from build123d import *

# Parameters (mm, degrees)
CROQUIS2_W              = 92
CROQUIS2_H              = 62
SALIENTE_EXTRUIR1_DEPTH = 8
CROQUIS3_W              = 89
CROQUIS3_H              = 59
CORTAR_EXTRUIR1_DEPTH   = 2
CROQUIS4_W              = 87
CROQUIS4_H              = 57
CORTAR_EXTRUIR2_DEPTH   = 3
CROQUIS5_W              = 10
CROQUIS5_H              = 53.632525493
CORTAR_EXTRUIR3_DEPTH   = 1
CORTAR_EXTRUIR4_REACH   = 57.696
CROQUIS6_W              = 15
CROQUIS6_H              = 10
CROQUIS7_R              = 5
CORTAR_EXTRUIR5_DEPTH   = 56.794264938
REDONDEO1_R             = 5
CROQUIS9_W              = 2.5
CROQUIS9_H              = 17.009234147
CROQUIS9_H_2            = 13.999979608
CROQUIS9_H_3            = 14.150072655
CROQUIS9_W_2            = 9.965409089
CROQUIS9_H_4            = 2.5
CROQUIS9_W_3            = 7.294458122
CROQUIS9_W_4            = 7.420347284
CROQUIS9_W_5            = 5
CORTAR_EXTRUIR7_DEPTH   = 2
CROQUIS10_R             = 1.492354092
CROQUIS10_R_2           = 1.54105633
CROQUIS10_R_3           = 1.454647155
CROQUIS10_R_4           = 1.436117112
CORTAR_EXTRUIR8_DEPTH   = 56.695601345
CORTAR_EXTRUIR9_REACH   = 99.411
CROQUIS11_W             = 15
CROQUIS11_H             = 8
CROQUIS12_W             = 50.407466657
CROQUIS12_H             = 2
CORTAR_EXTRUIR10_DEPTH  = 2.5
CROQUIS13_W             = 52.657281968
CROQUIS13_H             = 2
CORTAR_EXTRUIR11_DEPTH  = 2.5


with BuildPart() as part:
    # Croquis2 → Saliente-Extruir1 (new body)
    with BuildSketch(Plane(origin=(0, 0, 0), x_dir=(1, 0, 0), z_dir=(0, 1, 0))):
        Rectangle(CROQUIS2_W, CROQUIS2_H)
    extrude(amount=SALIENTE_EXTRUIR1_DEPTH)

    # Croquis3 → Cortar-Extruir1 (cut)
    with BuildSketch(Plane(origin=(0, 8, 0), x_dir=(1, 0, 0), z_dir=(0, 1, 0))):
        Rectangle(CROQUIS3_W, CROQUIS3_H)
    extrude(amount=-CORTAR_EXTRUIR1_DEPTH, mode=Mode.SUBTRACT)

    # Croquis4 → Cortar-Extruir2 (cut)
    with BuildSketch(Plane(origin=(0, 6, 0), x_dir=(1, 0, 0), z_dir=(0, 1, 0))):
        Rectangle(CROQUIS4_W, CROQUIS4_H)
    extrude(amount=-CORTAR_EXTRUIR2_DEPTH, mode=Mode.SUBTRACT)

    # Croquis5 → Cortar-Extruir3 (cut)
    with BuildSketch(Plane(origin=(0, 3, 0), x_dir=(1, 0, 0), z_dir=(0, 1, 0))):
        with Locations((-37, 0.183737253)):
            Rectangle(CROQUIS5_W, CROQUIS5_H)
    extrude(amount=-CORTAR_EXTRUIR3_DEPTH, mode=Mode.SUBTRACT)

    # Cortar-Extruir4: up to this face of the body (flat: up to its plane)
    cortar_extruir4_end = Plane(part.part.faces().sort_by_distance((-37, 2, -0.183737254))[0])
    # Croquis6 → Cortar-Extruir4 (cut, up to the picked face)
    with BuildSketch(Plane(origin=(0, 5, 0), x_dir=(1, 0, 0), z_dir=(0, 1, 0)), mode=Mode.PRIVATE) as cortar_extruir4_sk1:
        with Locations((38.5, 0)):
            Rectangle(CROQUIS6_W, CROQUIS6_H)
    cortar_extruir4_tool1 = split(extrude(cortar_extruir4_sk1.sketch, amount=-CORTAR_EXTRUIR4_REACH, mode=Mode.PRIVATE), bisect_by=cortar_extruir4_end, keep=Keep.BOTH, mode=Mode.PRIVATE)
    add(cortar_extruir4_tool1.solids().sort_by(Axis((38.5, 5, 0), (0, -1, 0)))[0], mode=Mode.SUBTRACT)

    # Croquis7 → Cortar-Extruir5 (cut, through all)
    with BuildSketch(Plane(origin=(0, 2, 0), x_dir=(1, 0, 0), z_dir=(0, 1, 0))):
        with Locations((46, 0)):
            Circle(CROQUIS7_R)
    extrude(amount=-CORTAR_EXTRUIR5_DEPTH, mode=Mode.SUBTRACT)

    # Redondeo1
    # the kernel refuses this fillet: 5 mm, written as the material it takes off along each edge
    with BuildSketch(Plane(origin=(46, 2, 0), x_dir=(0.9999950652018581, 0, -0.00314158748587981), z_dir=(0.00314158748587981, 0, 0.9999950652018581))) as redondeo1_piece_1_section:
        with BuildLine():
            CenterArc((9, -5), REDONDEO1_R, 90, 53.130102354)
            Line((9, 0), (5, 0))
            Line((5, 0), (5, -2))
        make_face()
    redondeo1_piece_1 = revolve(axis=Axis((46, 2, 0), (0, 1, 0)), revolution_arc=359.64, mode=Mode.PRIVATE)
    redondeo1_piece_1 = split(redondeo1_piece_1, bisect_by=Plane(origin=(39.240540113, 1.481080227, 5), z_dir=(0, 0, -1)), keep=Keep.TOP, mode=Mode.PRIVATE)
    redondeo1_piece_1 = split(redondeo1_piece_1, bisect_by=Plane(origin=(39.240540113, 1.481080227, -5), z_dir=(0, 0, 1)), keep=Keep.TOP, mode=Mode.PRIVATE)
    add(redondeo1_piece_1, mode=Mode.SUBTRACT)

    # Croquis9 → Cortar-Extruir7 (cut)
    with BuildSketch(Plane(origin=(0, 8, 0), x_dir=(1, 0, 0), z_dir=(0, 1, 0))):
        with Locations((-44.75, -18.601084438)):
            Rectangle(CROQUIS9_W, CROQUIS9_H)
        with Locations((-44.75, 0.477589339)):
            Rectangle(CROQUIS9_W, CROQUIS9_H_2)
        with Locations((-44.75, 18.476544129)):
            Rectangle(CROQUIS9_W, CROQUIS9_H_3)
        with Locations((31.175863948, 29.75)):
            Rectangle(CROQUIS9_W_2, CROQUIS9_H_4)
        with Locations((16.194930406, 29.75)):
            Rectangle(CROQUIS9_W_3, CROQUIS9_H_4)
        with Locations((2.577919336, 29.75)):
            Rectangle(CROQUIS9_W_4, CROQUIS9_H_4)
        with Locations((-11.725767222, 29.75)):
            Rectangle(CROQUIS9_W_5, CROQUIS9_H_4)
    extrude(amount=-CORTAR_EXTRUIR7_DEPTH, mode=Mode.SUBTRACT)

    # Croquis10 → Cortar-Extruir8 (cut, through all)
    with BuildSketch(Plane(origin=(0, 3, 0), x_dir=(1, 0, 0), z_dir=(0, 1, 0))):
        with Locations(Location((39.042237476, -25.238379945, 0), (0, 0, 270))):
            Circle(CROQUIS10_R)
        with Locations(Location((39.042237476, 23.410831917, 0), (0, 0, 270))):
            Circle(CROQUIS10_R_2)
        with Locations(Location((-19.081524932, 23.410831917, 0), (0, 0, 270))):
            Circle(CROQUIS10_R_3)
        with Locations(Location((-19.081524932, -25.238379945, 0), (0, 0, 270))):
            Circle(CROQUIS10_R_4)
    extrude(amount=-CORTAR_EXTRUIR8_DEPTH, mode=Mode.SUBTRACT)

    # Cortar-Extruir9: up to this face of the body (flat: up to its plane)
    cortar_extruir9_end = Plane(part.part.faces().sort_by_distance((31, 2.5, 0))[0])
    # Croquis11 → Cortar-Extruir9 (cut, up to the picked face)
    with BuildSketch(Plane(origin=(46, 0, 0), x_dir=(0, 0, -1), z_dir=(1, 0, 0)), mode=Mode.PRIVATE) as cortar_extruir9_sk1:
        with Locations((0, 4)):
            Rectangle(CROQUIS11_W, CROQUIS11_H)
    cortar_extruir9_tool1 = split(extrude(cortar_extruir9_sk1.sketch, amount=-CORTAR_EXTRUIR9_REACH, mode=Mode.PRIVATE), bisect_by=cortar_extruir9_end, keep=Keep.BOTH, mode=Mode.PRIVATE)
    add(cortar_extruir9_tool1.solids().sort_by(Axis((46, 4, 0), (-1, 0, 0)))[0], mode=Mode.SUBTRACT)

    # Croquis12 → Cortar-Extruir10 (cut)
    with BuildSketch(Plane(origin=(0, 0, -31), x_dir=(-1, 0, 0), z_dir=(0, 0, -1))):
        with Locations((-10.977966106, 7)):
            Rectangle(CROQUIS12_W, CROQUIS12_H)
    extrude(amount=-CORTAR_EXTRUIR10_DEPTH, mode=Mode.SUBTRACT)

    # Croquis13 → Cortar-Extruir11 (cut)
    with BuildSketch(Plane.ZY.offset(46)):
        with Locations((0.777060527, 7)):
            Rectangle(CROQUIS13_W, CROQUIS13_H)
    extrude(amount=-CORTAR_EXTRUIR11_DEPTH, mode=Mode.SUBTRACT)


solid = part.part
Geometry: final body of the model. Coordinates: model frame, mm. A direction names the side the tool comes from. Coordinates: 2 decimals unless noted, no trailing zeros. Loops run counter-clockwise (first coordinate to the right, second up) from the corner with the lowest first, then second, coordinate; pieces in that order, holes last. Notation, with made-up numbers: M 42,8 L 53,8 A24 ccw 53,31 Z; hole C -7.5,6.25 d4. An arc over 180 degrees is marked long. One line per item, written item: value. Start each with the question number.
1) Material intervals for L1, parallel to X at y = 4.5, z = 20; L2, parallel to Z at x = -39.5, y = 4; L3, parallel to Y at x = 30, z = -5, sorted ascending. Write a range as from..to.
2) Pin query (flat end, axial travel): P1, Ø8, axis at x = 6, z = 21, coming from the +Y side; P2, Ø0.5, axis at y = 2.5, z = -2.5, coming from the +X side. Return the tip coordinate at first contact, or that it passes through.
3) Cut plane D-D (z = -2.5). Return loops of the section in (x, y), then the cut area to 4 significant figures.
4) Cut plane B-B (x = -36). Return loops of the section in (y, z), then the cut area to 3 significant figures.
5) Reachability of faces 4 (the flat face through (-43.5, 5, 0)), 5 (the flat face through (40, 2, -7.5)), 6 (the flat face through (-31, 8, -30)) from +Z, -Z, +X, -X, +Y, -Y: full face, straight path, thin tool, end or side. Return the list, or none.
6) Draft query along X for faces 1 (the flat face through (0, 8, 30)), 2 (the flat face through (-44.5, 7, -27)), 3 (the flat face through (31, 2, 0)). Return one class per face: released by +X, released by -X, zero draft, split by the parting line, or undercut.
7) Cut plane C-C (y = 4.75). Return loops of the section in (x, z).
8) Cut plane A-A (z = 19). Return loops of the section in (x, y), then the cut area to 3 significant figures.
Evaluation:
1. L1: -46..-43.5, 43.5..46
1. L2: -31..-28.5, 28.5..31
1. L3: 0..3
2. P1: y = 3
2. P2: x = 31
3. outline: M -46,0 L 31,0 L 31,3 L -32,3 L -32,2 L -42,2 L -42,3 L -43.5,3 L -43.5,6 L -46,6 Z
3. area: 228.5 mm^2
4. outline: M 0,-31 L 8,-31 L 8,-29.5 L 6,-29.5 L 6,-28.5 L 3,-28.5 L 3,-27 L 2,-27 L 2,26.63 L 3,26.63 L 3,28.5 L 6,28.5 L 6,29.5 L 8,29.5 L 8,31 L 0,31 Z
4. area: 153 mm^2
5. face 4: +Y
5. face 5: +X, +Y, -Y
5. face 6: +Z, -Z, +X, -X, +Y
6. face 1: zero draft
6. face 2: undercut
6. face 3: released by +X
7. outline: M -46,-31 L 46,-31 L 46,-7.5 L 43.5,-7.5 L 43.5,-28.5 L -43.5,-28.5 L -43.5,28.5 L 43.5,28.5 L 43.5,7.5 L 46,7.5 L 46,31 L -46,31 Z
8. outline: M -46,0 L 46,0 L 46,8 L 44.5,8 L 44.5,6 L 43.5,6 L 43.5,3 L -32,3 L -32,2 L -42,2 L -42,3 L -43.5,3 L -43.5,6 L -46,6 Z
8. area: 284 mm^2
